```python
from build123d import *

# Parameters (mm, degrees)
BOSS_EXTRUDE1_START = 8
BOSS_EXTRUDE1_DEPTH = 8
BOSS_EXTRUDE2_START = 7
BOSS_EXTRUDE2_DEPTH = 12
BOSS_EXTRUDE3_DEPTH = 25


with BuildPart() as part:
    # Sketch1 → Boss-Extrude1 (new body)
    with BuildSketch(Plane.XY.offset(BOSS_EXTRUDE1_START)):
        with BuildLine():
            Line((74.83730752, 9.983544534), (57.235944241, 8.551998103))
            Line((57.235944241, 8.551998103), (51.260118774, 2.106214182))
            ThreePointArc((51.260118774, 2.106214182), (44.723252789, 3.063686722), (47.994339706, 8.803665899))
            Line((47.994339706, 8.803665899), (74.756243624, 10.980253441))
            ThreePointArc((74.756243624, 10.980253441), (80.9122, 6.963655259), (78.559251789, 0))
            Line((78.559251789, 0), (75.242626998, 0))
            ThreePointArc((75.242626998, 0), (80.238511438, 5.202826688), (74.83730752, 9.983544534))
        make_face()
        with BuildLine():
            Line((50.524737903, 2.783868204), (55.553573418, 8.241091684))
            ThreePointArc((55.553573418, 8.241091684), (55.569918893, 8.352685675), (55.471928941, 8.408527977))
            Line((55.471928941, 8.408527977), (48.075403602, 7.806956992))
            ThreePointArc((48.075403602, 7.806956992), (45.622088414, 3.501972609), (50.524737903, 2.783868204))
        make_face(mode=Mode.SUBTRACT)
    extrude(amount=BOSS_EXTRUDE1_DEPTH)



with BuildPart() as body_2:
    # Sketch1_5 → Boss-Extrude2 (new body)
    with BuildSketch(Plane.XY.offset(BOSS_EXTRUDE2_START)):
        with BuildLine():
            Line((124.883891422, 18.696355808), (92.855908874, 10.61849306))
            ThreePointArc((92.855908874, 10.61849306), (90.346819157, 4.780693613), (96.637825713, 3.88701016))
            Line((96.637825713, 3.88701016), (107.85561912, 13.370294626))
            Line((107.85561912, 13.370294626), (125.128445793, 17.726720227))
            ThreePointArc((125.128445793, 17.726720227), (136.260853893, 10.108944985), (127.329435135, 0))
            Line((127.329435135, 0), (127.329435135, -1))
            ThreePointArc((127.329435135, -1), (137.253233755, 10.232161094), (124.883891422, 18.696355808))
        make_face()
        with BuildLine():
            ThreePointArc((93.100463246, 9.648857479), (91.218645958, 5.270507894), (95.936900874, 4.600245304))
            Line((95.936900874, 4.600245304), (105.648911717, 12.813735076))
            Line((105.648911717, 12.813735076), (93.100463246, 9.648857479))
        make_face(mode=Mode.SUBTRACT)
    extrude(amount=BOSS_EXTRUDE2_DEPTH)


with BuildPart() as part_1:
    add(part.part)

    add(body_2.part)  # Boss-Extrude3 merges body 2
    # Sketch1_6 → Boss-Extrude3 (add)
    with BuildSketch(Plane.XY):
        Polygon((8.329435135, 0), (75.242626998, 0), (78.559251789, 0), (127.329435135, 0), (127.329435135, -1), (8.329435135, -1), align=None)
    extrude(amount=BOSS_EXTRUDE3_DEPTH)


solid = part_1.part
```
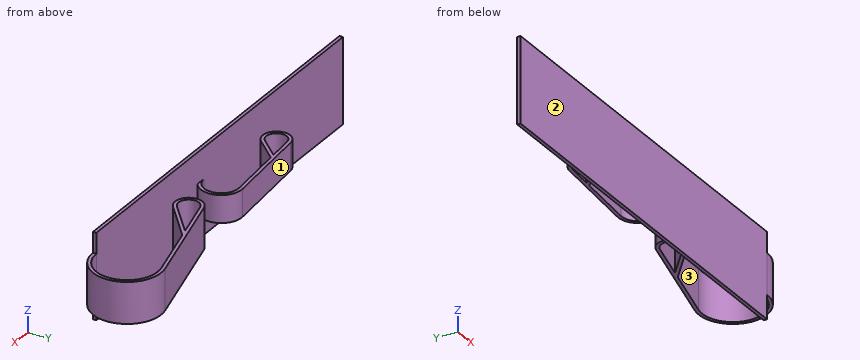
CAD build for the part. Positions are in the model's coordinates, mm. Face numbers are marked on the shaded views. Round coordinates to 2 decimals unless told otherwise and drop trailing zeros. Order: outer loops, then holes, each group sorted by start corner. A loop starts at its lowest first (then second) coordinate and runs counter-clockwise, first axis right, second up. Notation, with made-up numbers: (-25.5, 32.25) -> (-2.5, 32.25) arc R29 cw to (-2.5, 70.25) -> close; hole circle Ø7 at (-12.75, 36). An arc over 180 degrees is marked (long way). Write item = value, one per line.
(1) Cut at B-B (z = 9.5). Write the cut outline in (x, y).
Answers follow:
outline = (8.33, -1) -> (127.33, -1) arc R10 ccw (long way) to (124.88, 18.7) -> (92.86, 10.62) arc R4 ccw (long way) to (96.64, 3.89) -> (107.86, 13.37) -> (125.13, 17.73) arc R9 cw (long way) to (127.33, 0) -> (78.56, 0) arc R6 ccw to (74.76, 10.98) -> (47.99, 8.8) arc R4 ccw (long way) to (51.26, 2.11) -> (57.24, 8.55) -> (74.84, 9.98) arc R5 cw (long way) to (75.24, 0) -> (8.33, 0) -> close; hole (48.08, 7.81) arc R3 ccw (long way) to (50.52, 2.78) -> (55.55, 8.24) arc R0.1 ccw to (55.47, 8.41) -> close; hole (93.1, 9.65) arc R3 ccw (long way) to (95.94, 4.6) -> (105.65, 12.81) -> close
(2) Cut at A-A (x = 72.5). Write the cut outline in (y, z), plus the area to 3 significant figures.
Answers follow:
outline = (-1, 0) -> (0, 0) -> (0, 25) -> (-1, 25) -> close; (9.79, 8) -> (10.8, 8) -> (10.8, 16) -> (9.79, 16) -> close
area = 33.0 mm²
(3) Cut at C-C (x = 23). Write the cut outline in (y, z).
Answers follow:
outline = (-1, 0) -> (0, 0) -> (0, 25) -> (-1, 25) -> close
(4) Pull direction X, two halves, no side cores. Call the marked faces 1, 2 and 3: +X half, -X half, draft (parallel to the pull), parting line (faces both ways), or undercut.
Answers follow:
face_1 = -X half
face_2 = draft
face_3 = undercut
(5) Drill centre lines: L1, parallel to X at y = 1.25, z = 8.75; L2, parallel to Y at x = 45, z = 7.25; L3, parallel to X at y = 1.5, z = 15.5. Where is each one in solid material? Low to high.
Answers follow:
L1 = 46.51 to 50.13, 78.55 to 79.93, 131.91 to 133.65
L2 = -1 to 0
L3 = 46.08 to 50.55, 78.81 to 80.12, 132.3 to 133.94
(6) Flat gauge pins, fed straight in: P1, Ø12, axis at y = 3, z = 4.5, coming from the +X side; P2, Ø0.5, axis at y = -0.5, z = 2, coming from the +X side; P3, Ø4, axis at y = 13.5, z = 12.5, coming from the +X side; P4, Ø2, axis at x = 82.5, y = 2, coming from the -Z side. Where does each tip first touch, or does it go through?
Answers follow:
P1 = 137.31
P2 = 127.33
P3 = 137.01
P4 = through
